Autodesk Inventor part; units mm, degrees
ref_plane "YZ Plane" through (0, 0, 0) normal (1, 0, 0) x (0, 1, 0)
ref_plane "XZ Plane" through (0, 0, 0) normal (0, 1, 0) x (-1, 0, 0)
ref_plane "XY Plane" through (0, 0, 0) normal (0, 0, 1) x (1, 0, 0)
sketch "Эскиз1" plane through (0, 0, 0) normal (0, 1, 0) x (-1, 0, 0)
  line L0 (14.899, 13.3523) -> (-2.101, 13.3523)
  line L1 (-2.101, 13.3523) -> (-2.101, -11.6477)
  line L2 (-2.101, -11.6477) -> (14.899, -11.6477)
  line L3 (14.899, -11.6477) -> (14.899, 13.3523)
  point P0 (0, 0)
  dimension "d0" = 25
  dimension "d1" = 17
extrude "Выдавливание1" add sketch "Эскиз1" along normal blind 1
sketch "Эскиз2" plane through (0, 1, 0) normal (0, 1, 0) x (1, 0, 0)
  line L0 (-14.899, 11.6477) -> (-14.899, -13.3523) construction
  line L1 (2.101, -13.3523) -> (2.101, 11.6477) construction
  line L2 (-14.899, -13.3523) -> (2.101, 11.6477) construction
  line L3 (2.101, 11.6477) -> (-14.899, 11.6477) construction
  line L4 (-14.899, 11.6477) -> (2.101, -13.3523) construction
  line L5 (-13.899, -12.3523) -> (1.101, -12.3523) construction
  line L6 (1.101, -12.3523) -> (1.101, 10.6477) construction
  line L7 (1.101, 10.6477) -> (-13.899, 10.6477) construction
  line L8 (-13.899, 10.6477) -> (-13.899, -12.3523) construction
  line L9 (-13.899, -12.3523) -> (1.101, 10.6477) construction
  line L10 (1.101, -12.3523) -> (-13.899, 10.6477) construction
  circle A0 centre (-13.899, -12.3523) radius 0.5
  circle A1 centre (-13.899, 10.6477) radius 0.5
  circle A2 centre (1.101, 10.6477) radius 0.5
  circle A3 centre (1.101, -12.3523) radius 0.5
  circle A4 centre (-6.399, -0.8523) radius 5
  point P0 (0, 0)
  point P1 (-6.399, -0.8523)
  dimension "d4" = 23
  dimension "d5" = 15
  dimension "d6" = 1
  dimension "d7" = 10
extrude "Выдавливание2" add sketch "Эскиз2" along normal blind 1
properties part number "тест"
Here's how the part is built. I have some questions about the finished solid (model axes, mm). A direction names the side the tool comes from. Give positions to 0.01 mm unless a question says otherwise; leave off trailing zeros. Write each loop counter-clockwise with the first axis right and the second up, starting at its lowest first coordinate (ties: lowest second). Pieces come first, ordered by that corner, then holes.
(1) Imagine slicing it at A-A, the plane y = 1.45. Write out the boundary of the cut face in (x, z).
Output values:
outline: circle Ø1 at (-13.9, -10.65); circle Ø1 at (-13.9, 12.35); circle Ø10 at (-6.4, 0.85); circle Ø1 at (1.1, -10.65); circle Ø1 at (1.1, 12.35)
(2) Imagine slicing it at D-D, the plane x = -1. Write out the boundary of the cut face in (y, z).
Output values:
outline: (0, -11.65) - (1, -11.65) - (1, 13.35) - (0, 13.35) - close
(3) Thinking about a two-plate mould opening in Z: for faces 1 (the face through (-6.3, 0.5, -11.648)), 2 (the face through (-13.9, 2, -10.7)), 3 (the face through (1.33, 1.49, -11.09)), which applies, pulls with the +Z half, pulls with the -Z half, needs draft (parallel to the pull), parting line crosses it, or undercut?
Output values:
face 1: pulls with the -Z half
face 2: needs draft
face 3: undercut
(4) If I drill on L1, parallel to Y at x = -7.75, z = -9.5; L2, parallel to Z at x = -14, y = 1.4; L3, parallel to Z at x = -10.5, y = 1.65, over which ranges is the centre line in solid material (lowest first)?
Output values:
L1: y = 0 to 1
L2: z = -11.14 to -10.16, 11.86 to 12.84
L3: z = -2.01 to 3.71
(5) Imagine slicing it at B-B, the plane x = -5.5. Write out the boundary of the cut face in (y, z).
Output values:
outline: (0, -11.65) - (1, -11.65) - (1, -4.07) - (2, -4.07) - (2, 5.77) - (1, 5.77) - (1, 13.35) - (0, 13.35) - close
(6) On a 3-axis mill with a long thin cutter (end or side, diameter ignored), from which of +Z, -Z, +X, -X, +Y, -Y can I reach the whole of each face in a straight line? I mean faces 4 (the face through (-14.296, 1.493, -10.952)), 5 (the face through (1.1, 2, -10.7)). Say none if no direction works.
Output values:
face 4: +Y
face 5: +Z, -Z, +X, -X, +Y
(7) Will this pin go through, and if not, where does the flat tip stop? pin 1 (10 mm diameter, centred on x = -5, z = 11, fed in from +Y).
Output values:
pin 1: stops at y = 1
(8) Imagine slicing it at C-C, the plane z = 5.25. Write out the boundary of the cut face in (x, y).
Output values:
outline: (-14.9, 0) - (2.1, 0) - (2.1, 1) - (-4.02, 1) - (-4.02, 2) - (-8.78, 2) - (-8.78, 1) - (-14.9, 1) - close
